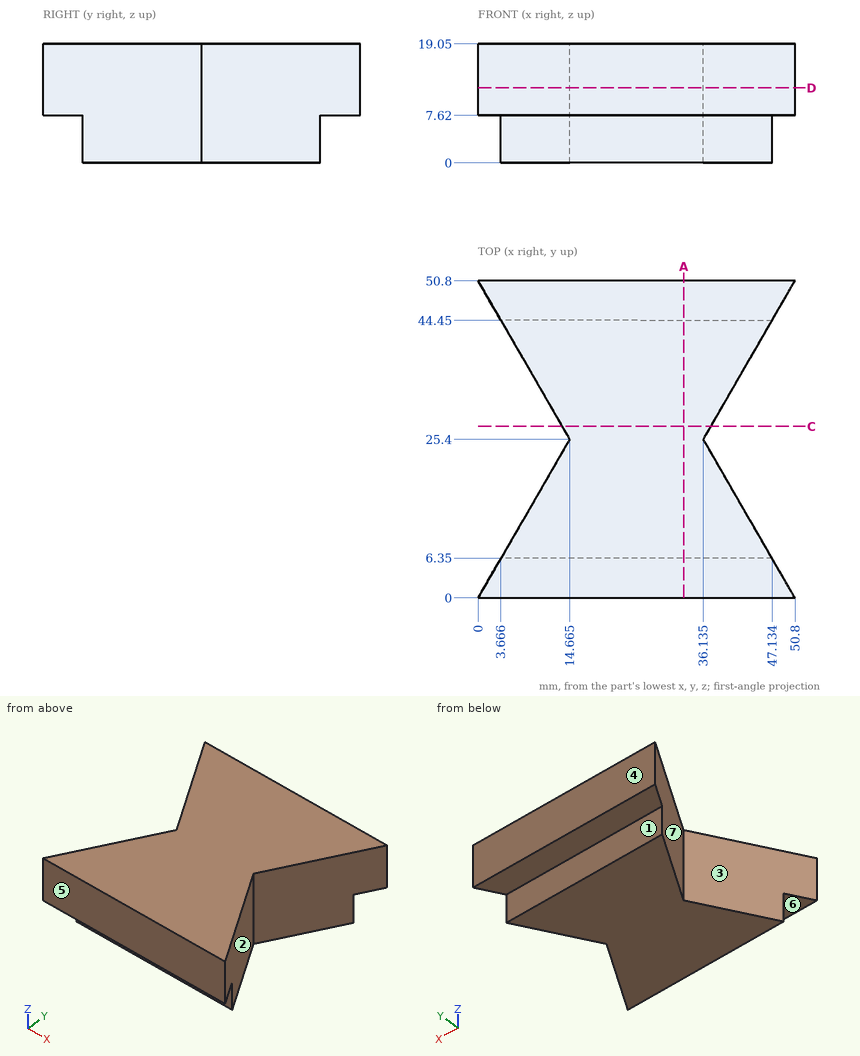
Print and shaded views of the part. All mm, measured from the part's lowest x, y and z. A direction names the side the tool comes from. Coordinates: 2 decimals unless noted, no trailing zeros. Loops run counter-clockwise (first coordinate to the right, second up) from the corner with the lowest first, then second, coordinate; pieces in that order, holes last. Notation, with made-up numbers: (42, 35.5) - (74, 35.5) arc R29 cw to (74, 64.5) - close; hole circle Ø3 at (-22, 0). An arc over 180 degrees is marked (long way). Write item = value, one per line. Start each with the question number.
Item 1: 3-axis set-ups, long thin cutter, end or side, ignore diameter. For the marked faces 1, 2 and 3: which of +Z, -Z, +X, -X, +Y, -Y reach the whole face in a straight line?
Item 2: Saw through at A-A, the plane x = 33. List the corners of the cut face in (y, z).
Item 3: Drop flat-ended pins along their axis: pin 1 Ø6 at (x, y) = (32, 29) entering from -Z; pin 2 Ø1.9 at (x, y) = (37, 3) entering from -Z; pin 3 Ø2 at (y, z) = (23, 16.5) entering from -X; pin 4 Ø6 at (x, z) = (29.5, 4) entering from +Y. Give the stop position or say it passes through.
Item 4: Wall check: probe 1 along Z at (x, y) = (15, 5.5); probe 2 along Y at (x, z) = (46, 16) (1 decimal); probe 3 along Y at (x, z) = (17, 2.25). Give the ranges that are in metal, low to high. Write a range as [from, to].
Item 5: Saw through at D-D, the plane z = 12. List the corners of the cut face in (x, y) (1 decimal).
Item 6: Pull direction Y, two halves, no side cores. Call the marked faces 4, 5, 6 and 7: +Y half, -Y half, draft (parallel to the pull), parting line (faces both ways), or undercut.
Item 7: Saw through at C-C, the plane y = 27.5. List the corners of the cut face in (x, z).
Answers:
q1.face_1 = -Z, +X, -X, +Y
q1.face_2 = +Z, -Z, +X
q1.face_3 = +Z, -Z, -X
q2.outline = (0, 7.62) - (6.35, 7.62) - (6.35, 0) - (44.45, 0) - (44.45, 7.62) - (50.8, 7.62) - (50.8, 19.05) - (0, 19.05) - close
q3.pin_1 = 0
q3.pin_2 = 7.62
q3.pin_3 = 12.7
q3.pin_4 = 44.45
q4.probe_1 = [7.62, 19.05]
q4.probe_2 = [0, 8.3], [42.5, 50.8]
q4.probe_3 = [6.35, 44.45]
q5.outline = (0, 0) - (50.8, 0) - (36.1, 25.4) - (50.8, 50.8) - (0, 50.8) - (14.7, 25.4) - close
q6.face_4 = +Y half
q6.face_5 = -Y half
q6.face_6 = draft
q6.face_7 = undercut
q7.outline = (13.45, 0) - (37.35, 0) - (37.35, 19.05) - (13.45, 19.05) - close
